Input: part model. Units: mm. Frame: model coordinates. A direction names the side the tool comes from. Round coordinates to 2 decimals unless told otherwise and drop trailing zeros. Loops run counter-clockwise (first coordinate to the right, second up) from the corner with the lowest first, then second, coordinate; pieces in that order, holes last. Notation, with made-up numbers: M 31.5,-8 L 58.5,-8 A29 cw 58.5,30 Z; hole C 17.25,85.5 d2. An arc over 180 degrees is marked long. Use one line per item in the form item = value. Start each with the question number.
Q1. Access query for faces 4 (the flat face through (0, 5, 0)), 5 (the flat face through (-4.11, 2.41, 92.33)). Directions: +Z, -Z, +X, -X, +Y, -Y. A direction counts if a zero-diameter tool reaches every point of the face in a straight line with its end or side. Return the directions, or none.
Q2. Mould query, pull axis X, two halves, no side actions, for faces 1 (the flat face through (0, 4.762, 92)), 2 (the flat face through (0, 5, 182.118)), 3 (the cylindrical face through (-5.506, -24.796, 89.854)). Classes: pulls with the +X half, pulls with the -X half, needs draft (parallel to the pull), parting line crosses it, or undercut.
Q3. Section query B-B, the plane z = 30.5. Output: boundary loops of the cut face in (x, y), and give its area (3 significant figures).
Q4. Ray query, line 1 along Y through (x, z) = (1, 166); line 2 along X through (y, z) = (-1.5, 41); line 3 along Y through (x, z) = (3, 37.5). Return the intervals inside material, ascending.
Q5. Section query A-A, the plane x = 0. Output: boundary loops of the cut face in (y, z).
Q6. First-contact query: P1, Ø5, axis at y = -12, z = 148, coming from the -X side; P2, Ø1, axis at x = -13.5, z = 133.5, coming from the +Y side; P3, Ø2, axis at y = -18.5, z = 80, coming from the -X side; P4, Ø3, axis at y = 1, z = 124, coming from the -X side. Flat tips, straight axial feed; report the tip coordinate or a pass-through.
```python
from build123d import *

# Parameters (mm, degrees)
SKETCH1_R           = 25.4
BOSS_EXTRUDE1_DEPTH = 182.118
CUT_EXTRUDE1_DEPTH  = 183.118
FILLET1_R           = 5


with BuildPart() as part:
    # Sketch1 → Boss-Extrude1 (new body)
    with BuildSketch(Plane.XY):
        Circle(SKETCH1_R)
    extrude(amount=BOSS_EXTRUDE1_DEPTH)

    # Sketch2 → Cut-Extrude1 (cut, through all)
    with BuildSketch(Plane.XY.offset(182.118)):
        Polygon((5.499261314, 0), (2.749630657, 4.7625), (-2.749630657, 4.7625), (-5.499261314, 0), (-2.749630657, -4.7625), (2.749630657, -4.7625), align=None)
    extrude(amount=-CUT_EXTRUDE1_DEPTH, mode=Mode.SUBTRACT)

    # Fillet1
    fillet1_edges = [part.edges().sort_by_distance(p)[0] for p in [
        (-25.4, 0, 0),
        (-25.4, 0, 182.118),
    ]]
    fillet(fillet1_edges, radius=FILLET1_R)


solid = part.part
```
Results found:
q1.face_4 = -Z, +X, -X, +Y, -Y
q1.face_5 = +Z, -Z
q2.face_1 = undercut
q2.face_2 = needs draft
q2.face_3 = parting line crosses it
q3.outline = C 0,0 d50.8; hole M -5.5,0 L -2.75,-4.76 L 2.75,-4.76 L 5.5,0 L 2.75,4.76 L -2.75,4.76 Z
q3.area = 1,950 mm²
q4.line_1 = -25.38 to -4.76, 4.76 to 25.38
q4.line_2 = -25.36 to -4.63, 4.63 to 25.36
q4.line_3 = -25.22 to -4.33, 4.33 to 25.22
q5.outline = M -25.4,5 A5 ccw -20.4,0 L -4.76,0 L -4.76,182.12 L -20.4,182.12 A5 ccw -25.4,177.12 Z; M 4.76,0 L 20.4,0 A5 ccw 25.4,5 L 25.4,177.12 A5 ccw 20.4,182.12 L 4.76,182.12 Z
q6.P1 = -23.56
q6.P2 = 21.82
q6.P3 = -18.41
q6.P4 = -25.4
